```python
from build123d import *

# Parameters (mm, degrees)
F1_DEPTH = 3


with BuildPart() as f1:
    # F0 (on Front) → F1 (new body)
    with BuildSketch(Plane.XZ):
        with BuildLine():
            Line((-70, 0), (-70, -10))
            Line((-70, -10), (-51.964102, -10))
            Line((-51.964102, -10), (-48.598076, -4.169873))
            Line((-48.598076, -4.169873), (-46, -5.669873))
            Line((-46, -5.669873), (-48.5, -10))
            Line((-48.5, -10), (-1.964102, -10))
            Line((-1.964102, -10), (1.401924, -4.169873))
            Line((1.401924, -4.169873), (4, -5.669873))
            Line((4, -5.669873), (1.5, -10))
            Line((1.5, -10), (48.035898, -10))
            Line((48.035898, -10), (51.401924, -4.169873))
            Line((51.401924, -4.169873), (54, -5.669873))
            Line((54, -5.669873), (51.5, -10))
            Line((51.5, -10), (70, -10))
            Line((70, -10), (70, 0))
            ThreePointArc((70, 0), (67.071068, 7.071068), (60, 10))
            Line((60, 10), (-60, 10))
            ThreePointArc((-60, 10), (-67.071068, 7.071068), (-70, 0))
        make_face()
    extrude(amount=F1_DEPTH)


solid = f1.part
```
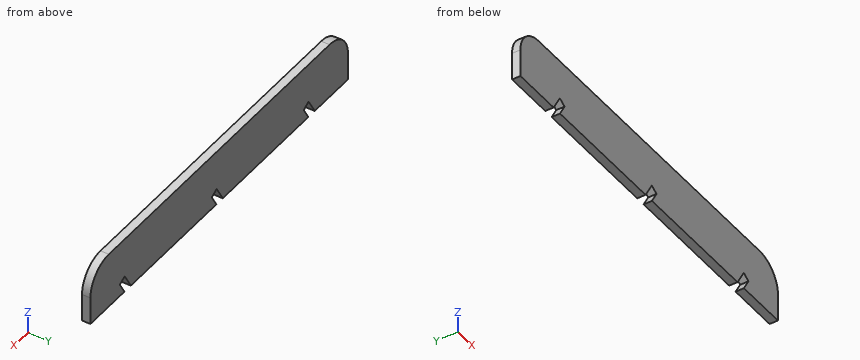
Geometry: final body of the model. Coordinates: model frame, mm. Give positions to 0.01 mm unless a question says otherwise; leave off trailing zeros. Write each loop counter-clockwise with the first axis right and the second up, starting at its lowest first coordinate (ties: lowest second). Pieces come first, ordered by that corner, then holes.
1. Line query: probe 1 along X at (y, z) = (-2.25, -8.5); probe 2 along X at (y, z) = (-2, -5.5); probe 3 along X at (y, z) = (-0.9, 0.75). Output: solid intervals per line, ascending.
2. Section query A-A, the plane y = -0.6. Return loops of the section in (x, z).
3. Section query B-B, the plane z = 5.5. Return loops of the section in (x, y).
Computed:
1. probe 1: x = -70 to -51.1, -47.63 to -1.1, 2.37 to 48.9, 52.37 to 70
1. probe 2: x = -70 to -49.37, -46.29 to 0.63, 3.71 to 50.63, 53.71 to 70
1. probe 3: x = -69.97 to 69.97
2. outline: (-70, -10) - (-51.96, -10) - (-48.6, -4.17) - (-46, -5.67) - (-48.5, -10) - (-1.96, -10) - (1.4, -4.17) - (4, -5.67) - (1.5, -10) - (48.04, -10) - (51.4, -4.17) - (54, -5.67) - (51.5, -10) - (70, -10) - (70, 0) arc R10 ccw to (60, 10) - (-60, 10) arc R10 ccw to (-70, 0) - close
3. outline: (-68.35, -3) - (68.35, -3) - (68.35, 0) - (-68.35, 0) - close
